Geometry check sheet. Reference: the model listing, model coordinates, mm. A direction names the side the tool comes from. Coordinates: 2 decimals unless noted, no trailing zeros. Loops run counter-clockwise (first coordinate to the right, second up) from the corner with the lowest first, then second, coordinate; pieces in that order, holes last.
from build123d import *

# Parameters (mm, degrees)
SKETCH1_W                                            = 97
SKETCH1_H                                            = 292
BOSS_EXTRUDE1_DEPTH                                  = 18
SKETCH2_W                                            = 27
SKETCH2_H                                            = 20
SKETCH2_H_2                                          = 22
CUT_EXTRUDE1_DEPTH                                   = 155.894318811
SKETCH3_W                                            = 97
SKETCH3_H                                            = 332
BOSS_EXTRUDE2_DEPTH                                  = 15
CHAMFER1_SIZE                                        = 5
FILLET1_R                                            = 5
CUT_EXTRUDE2_DEPTH                                   = 174.874236159
CBORE_FOR_M4_HEXAGON_SOCKET_HEAD_CAP_SCR_D           = 4.5
CBORE_FOR_M4_HEXAGON_SOCKET_HEAD_CAP_SCR_CBORE_D     = 8
CBORE_FOR_M4_HEXAGON_SOCKET_HEAD_CAP_SCR_CBORE_DEPTH = 8
M4_CLEARANCE_HOLE1_D                                 = 4.5
CBORE_FOR_M6_SLOTTED_CHEESE_HEAD_SCREWS2_D           = 6.6
CBORE_FOR_M6_SLOTTED_CHEESE_HEAD_SCREWS2_CBORE_D     = 11
CBORE_FOR_M6_SLOTTED_CHEESE_HEAD_SCREWS2_CBORE_DEPTH = 6.8
CHAMFER2_SIZE                                        = 4
CUT_EXTRUDE3_DEPTH                                   = 177.060358968
FILLET4_R                                            = 8
SKETCH13_W                                           = 6
SKETCH13_H                                           = 175
CUT_EXTRUDE4_DEPTH                                   = 15
FILLET5_R                                            = 3


with BuildPart() as part:
    # Sketch1 → Boss-Extrude1 (new body)
    with BuildSketch(Plane.XY):
        Rectangle(SKETCH1_W, SKETCH1_H)
    extrude(amount=BOSS_EXTRUDE1_DEPTH)

    # Sketch2 → Cut-Extrude1 (cut, through all)
    with BuildSketch(Plane(origin=(0, 0, 0), x_dir=(-1, 0, 0), z_dir=(0, 0, -1))):
        with Locations((-35, -136)):
            Rectangle(SKETCH2_W, SKETCH2_H)
        with Locations((-35, 135)):
            Rectangle(SKETCH2_W, SKETCH2_H_2)
    extrude(amount=-CUT_EXTRUDE1_DEPTH, mode=Mode.SUBTRACT)

    # Sketch3 → Boss-Extrude2 (add)
    with BuildSketch(Plane.XY.offset(18)):
        Rectangle(SKETCH3_W, SKETCH3_H)
    extrude(amount=BOSS_EXTRUDE2_DEPTH)

    # Chamfer1
    chamfer1_edges = [part.edges().sort_by_distance(p)[0] for p in [
        (48.5, -126, 9),
        (21.5, -146, 9),
        (48.5, 124, 9),
        (21.5, 146, 9),
        (-48.5, 146, 9),
        (-48.5, -146, 9),
    ]]
    chamfer(chamfer1_edges, length=CHAMFER1_SIZE)

    # Fillet1
    fillet1_edges = [part.edges().sort_by_distance(p)[0] for p in [
        (21.5, -126, 9),
        (21.5, 124, 9),
    ]]
    fillet(fillet1_edges, radius=FILLET1_R)

    # Sketch4 → Cut-Extrude2 (cut, through all)
    with BuildSketch(Plane(origin=(0, 0, 18), x_dir=(-1, 0, 0), z_dir=(0, 0, -1))):
        with BuildLine():
            Line((0.9, -148), (15.9, -148))
            ThreePointArc((15.9, -148), (22.9, -155), (15.9, -162))
            Line((15.9, -162), (0.9, -162))
            ThreePointArc((0.9, -162), (-6.1, -155), (0.9, -148))
        make_face()
    extrude(amount=-CUT_EXTRUDE2_DEPTH, mode=Mode.SUBTRACT)

    # CBORE for M4 Hexagon socket head cap screws1 (through all)
    with Locations(Plane.XY.offset(33)):
        with Locations((-43.5, -141), (-43.5, -131), (16.5, -131), (16.5, -141), (16.5, 141), (16.5, 131), (-43.5, 131), (-43.5, 141), (22.5, -121), (34.5, -121), (22.5, -106), (34.5, -106), (34.5, 104), (22.5, 104), (34.5, 119), (22.5, 119)):
            CounterBoreHole(CBORE_FOR_M4_HEXAGON_SOCKET_HEAD_CAP_SCR_D / 2, CBORE_FOR_M4_HEXAGON_SOCKET_HEAD_CAP_SCR_CBORE_D / 2, CBORE_FOR_M4_HEXAGON_SOCKET_HEAD_CAP_SCR_CBORE_DEPTH)

    # M4 Clearance Hole1 (through all)
    with Locations(Plane.XY.offset(33)):
        with Locations((28.5, -96), (-13.5, -116), (28.5, 94), (-13.5, 118)):
            Hole(M4_CLEARANCE_HOLE1_D / 2)

    # CBORE for M6 Slotted cheese head screws2 (through all)
    with Locations(Plane.XY.offset(33)):
        with Locations((-38.5, 156), (-38.5, -156), (38.5, -156), (38.5, 156)):
            CounterBoreHole(CBORE_FOR_M6_SLOTTED_CHEESE_HEAD_SCREWS2_D / 2, CBORE_FOR_M6_SLOTTED_CHEESE_HEAD_SCREWS2_CBORE_D / 2, CBORE_FOR_M6_SLOTTED_CHEESE_HEAD_SCREWS2_CBORE_DEPTH)

    # Chamfer2
    chamfer2_edges = [part.edges().sort_by_distance(p)[0] for p in [
        (-48.5, 166, 25.5),
        (-48.5, -166, 25.5),
        (48.5, -166, 25.5),
        (48.5, 166, 25.5),
    ]]
    chamfer(chamfer2_edges, length=CHAMFER2_SIZE)

    # Sketch12 → Cut-Extrude3 (cut, through all)
    with BuildSketch(Plane.XY.offset(33)):
        Polygon((-33.5, -105), (-33.5, 105), (-3.5, 105), (21.5, 80), (33.5, 80), (33.5, -80), (21.5, -80), (-3.5, -105), align=None)
    extrude(amount=-CUT_EXTRUDE3_DEPTH, mode=Mode.SUBTRACT)

    # Fillet4
    fillet4_edges = [part.edges().sort_by_distance(p)[0] for p in [
        (-33.5, 105, 16.5),
        (-3.5, 105, 16.5),
        (21.5, 80, 16.5),
        (33.5, 80, 16.5),
        (33.5, -80, 16.5),
        (21.5, -80, 16.5),
        (-3.5, -105, 16.5),
        (-33.5, -105, 16.5),
    ]]
    fillet(fillet4_edges, radius=FILLET4_R)

    # Sketch13 → Cut-Extrude4 (cut)
    with BuildSketch(Plane(origin=(0, 0, 0), x_dir=(-1, 0, 0), z_dir=(0, 0, -1))):
        with Locations((45.5, 0)):
            Rectangle(SKETCH13_W, SKETCH13_H)
    extrude(amount=-CUT_EXTRUDE4_DEPTH, mode=Mode.SUBTRACT)

    # Fillet5
    fillet5_edges = [part.edges().sort_by_distance(p)[0] for p in [
        (-42.5, -87.5, 7.5),
        (-42.5, 87.5, 7.5),
    ]]
    fillet(fillet5_edges, radius=FILLET5_R)


solid = part.part
1) Depth check by flat-ended pin: pin 1 (2.5 mm diameter, centred on x = -47, z = 10.5, fed in from +Y); pin 2 (7 mm diameter, centred on x = -43.5, y = -141, fed in from -Z); pin 3 (3 mm diameter, centred on x = 28.5, z = 9, fed in from +Y); pin 4 (9.5 mm diameter, centred on x = -17, z = 9, fed in from -Y). Enter the tip coordinate at first touch or a pass-through.
Data:
pin 1: stops at y = 143.75
pin 2: stops at z = 0
pin 3: stops at y = 124
pin 4: stops at y = -146
2) Mould release check, pull along Y, two halves, no side actions. Record for faces 1 (the flat face through (36, -123, 25)), 2 (the flat face through (-48.5, -2, 20)), 3 (the flat face through (-1, -166, 25)): +Y half, -Y half, draft (parallel to the pull), parting line (faces both ways), or undercut.
Data:
face 1: undercut
face 2: draft
face 3: -Y half
3) Section check B-B on z = 29. Count the separate pieces of the cut face and the enclosed holes in it, and give its area (3 significant figures).
Data:
separate pieces: 1
enclosed holes: 26
area: 17,800 mm2
4) Section check A-A on y = -39. Record the cut outline in (x, z).
Data:
outline: (-48.5, 15) - (-42.5, 15) - (-42.5, 0) - (-33.5, 0) - (-33.5, 33) - (-48.5, 33) - close; (33.5, 0) - (48.5, 0) - (48.5, 33) - (33.5, 33) - close
5) Material ranges on probe 1 along Y at (x, z) = (34.5, 8.75); probe 2 along Y at (x, z) = (-14, 9.5); probe 3 along Y at (x, z) = (38.5, 21), recorded low to high.
Data:
probe 1: y = -126 to -123.25, -118.75 to -108.25, -103.75 to 101.75, 106.25 to 116.75, 121.25 to 124
probe 2: y = -146 to -118.19, -113.81 to -105, 105 to 115.81, 120.19 to 146
probe 3: y = -166 to -159.3, -152.7 to 152.7, 159.3 to 166
6) Access from +Z, -Z, +X, -X, +Y, -Y to the whole of each face (thin tool, end or side, straight path). Record for faces 4 (the flat face through (-16, -105, 17)), 5 (the flat face through (-42.5, -1, 7)), 6 (the flat face through (24, 102, 25)), 7 (the flat face through (-44, 2, 33)).
Data:
face 4: +Z, -Z
face 5: -Z, -X
face 6: +Z
face 7: +Z, +X, -X, +Y, -Y
